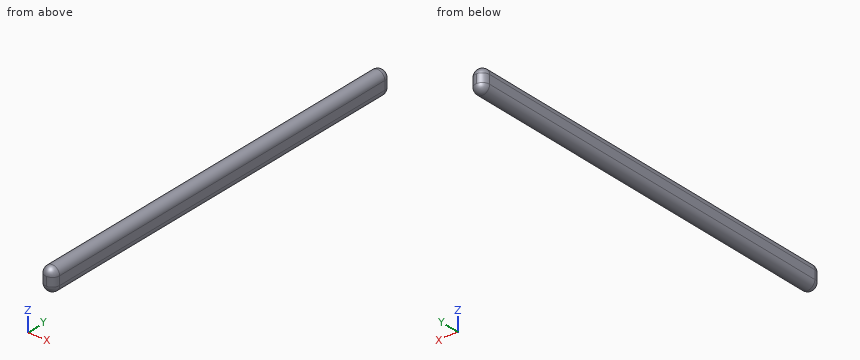
from build123d import *

# Parameters (mm, degrees)
BOSS_EXTRUDE1_DEPTH = 350
FILLET1_R           = 12.5


with BuildPart() as part:
    # Sketch2 → Boss-Extrude1 (new, symmetric)
    with BuildSketch(Plane(origin=(0, 0, 0), x_dir=(-1, 0, 0), z_dir=(0, 1, 0))):
        with BuildLine():
            Line((12.5, 7.5), (12.5, -7.5))
            ThreePointArc((12.5, -7.5), (0, -20), (-12.5, -7.5))
            Line((-12.5, -7.5), (-12.5, 7.5))
            ThreePointArc((-12.5, 7.5), (0, 20), (12.5, 7.5))
        make_face()
    extrude(amount=BOSS_EXTRUDE1_DEPTH, both=True)

    # Fillet1
    fillet1_edges = [part.edges().sort_by_distance(p)[0] for p in [
        (0, 350, -20),
        (-12.5, 350, 0),
        (0, 350, 20),
        (-12.5, -350, 0),
        (0, -350, -20),
        (12.5, -350, 0),
        (0, -350, 20),
        (12.5, 350, 0),
    ]]
    fillet(fillet1_edges, radius=FILLET1_R - 0.0001)  # a hair under: the kernel refuses the full size


solid = part.part
CAD build for the part. Positions are in the model's coordinates, mm. Round coordinates to 2 decimals unless told otherwise and drop trailing zeros. Loops run counter-clockwise (first coordinate to the right, second up) from the corner with the lowest first, then second, coordinate; pieces in that order, holes last.
(1) Wall check: line 1 along X through (y, z) = (137, 8.5); line 2 along Z through (x, y) = (0, -12.5); line 3 along X through (y, z) = (-304.5, 15). Give the ranges that are in metal, low to high.
(2) Cut at A-A (y = 58). Give the cut face in (x, z).
(3) Drop flat-ended pins along their axis: pin 1 (3 mm diameter, centred on x = 7, z = -14, fed in from -Y); pin 2 (10 mm diameter, centred on x = 6.5, z = 10, fed in from -Y); pin 3 (4 mm diameter, centred on x = -6, y = 74.5, fed in from +Z). Give the stop position or say it passes through.
Findings below:
1. line 1: x = -12.46 to 12.46
1. line 2: z = -20 to 20
1. line 3: x = -10 to 10
2. outline: (-12.5, -7.5) arc R12.5 ccw to (12.5, -7.5) - (12.5, 7.5) arc R12.5 ccw to (-12.5, 7.5) - close
3. pin 1: stops at y = -347.06
3. pin 2: stops at y = -349.84
3. pin 3: stops at z = 19.34
